Geometry check sheet. Reference: drawing and pictorial views, mm from the part's lowest x, y, z. Round coordinates to 2 decimals unless told otherwise and drop trailing zeros. Write each loop counter-clockwise with the first axis right and the second up, starting at its lowest first coordinate (ties: lowest second). Pieces come first, ordered by that corner, then holes.
Item 1: Section check A-A, the plane x = 66.5. Record the cut outline in (y, z).
Item 2: Section check B-B, the plane y = 62. Record the cut outline in (x, z), plus the area to 3 significant figures.
Item 3: Material ranges on line 1 along Y through (x, z) = (81.5, 1.2); line 2 along Y through (x, z) = (45.5, 2.4); line 3 along X through (y, z) = (87, 0.85), recorded low to high.
Item 4: Depth check by flat-ended pin: pin 1 (0.9 mm diameter, centred on y = 1, z = 2, fed in from -X); pin 2 (1.5 mm diameter, centred on x = 62.5, z = 1, fed in from +Y); pin 3 (0.9 mm diameter, centred on x = 61.5, z = 2, fed in from -Y). Enter the tip coordinate at first touch or a pass-through.
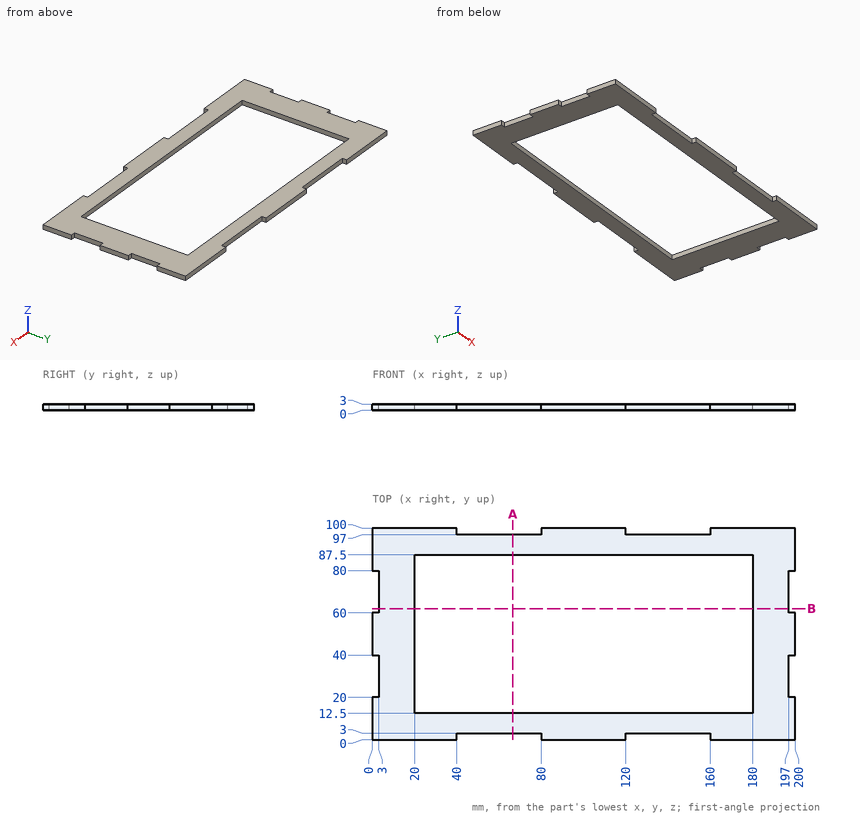
Values found:
1. outline: (3, 0) - (12.5, 0) - (12.5, 3) - (3, 3) - close; (87.5, 0) - (97, 0) - (97, 3) - (87.5, 3) - close
2. outline: (3, 0) - (20, 0) - (20, 3) - (3, 3) - close; (180, 0) - (197, 0) - (197, 3) - (180, 3) - close
2. area: 102 mm2
3. line 1: y = 0 to 12.5, 87.5 to 100
3. line 2: y = 3 to 12.5, 87.5 to 97
3. line 3: x = 0 to 20, 180 to 200
4. pin 1: stops at x = 0
4. pin 2: stops at y = 97
4. pin 3: stops at y = 3
